Autodesk Inventor part; units mm, degrees
ref_plane "YZ Plane" through (0, 0, 0) normal (1, 0, 0) x (0, 1, 0)
ref_plane "XZ Plane" through (0, 0, 0) normal (0, 1, 0) x (-1, 0, 0)
ref_plane "XY Plane" through (0, 0, 0) normal (0, 0, 1) x (1, 0, 0)
sketch "スケッチ1" plane through (0, 0, 0) normal (0, 0, 1) x (1, 0, 0)
  line L0 (4.5, 4.5) -> (-4.5, 4.5)
  line L1 (-4.5, 4.5) -> (-4.5, -4.5)
  line L2 (-4.5, -4.5) -> (4.5, -4.5)
  line L3 (4.5, -4.5) -> (4.5, 4.5)
  line L4 (4.5, 4.5) -> (-4.5, -4.5) construction
  line L5 (-4.5, 4.5) -> (4.5, -4.5) construction
  line L6 (-3.5, 3.5) -> (3.5, 3.5)
  line L7 (3.5, 3.5) -> (3.5, -3.5)
  line L8 (3.5, -3.5) -> (-3.5, -3.5)
  line L9 (-3.5, -3.5) -> (-3.5, 3.5)
  point P0 (0, 0)
  dimension "d0" = 9
  dimension "d1" = 9
  dimension "d2" = 1
extrude "押し出し1" add sketch "スケッチ1" along normal blind 79
sketch "スケッチ2" plane through (4.5, -4.5, 0) normal (1, 0, 0) x (0, 0, -1)
  circle A0 centre (-4.5, 4.5) radius 1.6
  circle A1 centre (-74.5, 4.5) radius 1.6
  line L0 (0, 0) -> (0, 9)
  point P0 (0, 4.5)
  point P1 (0, 4.5)
  dimension "d5" = 3.2
  dimension "d6" = 3.2
  dimension "d7" = 4.5
  dimension "d8" = 70
extrude "押し出し2" cut sketch "スケッチ2" against normal through all
sketch "スケッチ3" plane through (-4.5, 4.5, 0) normal (0, 1, 0) x (1, 0, 0)
  circle A0 centre (4.5, -14.5) radius 1.6
  circle A1 centre (4.5, -64.5) radius 1.6
  line L0 (9, 0) -> (0, 0)
  point P0 (4.5, 0)
  point P1 (4.5, 0)
  dimension "d11" = 3.2
  dimension "d12" = 3.2
  dimension "d13" = 50
  dimension "d14" = 14.5
extrude "押し出し3" cut sketch "スケッチ3" against normal through all
properties part number "ハンド_角柱2" material "アルミニウム 6061"
For this review, take the finished solid that the model builds, in its own axes (mm). A direction names the side the tool comes from. Coordinates: 2 decimals unless noted, no trailing zeros. Loops run counter-clockwise (first coordinate to the right, second up) from the corner with the lowest first, then second, coordinate; pieces in that order, holes last. Notation, with made-up numbers: (-26, 3) -> (33, 3) arc R29 cw to (33, 25) -> close; hole circle Ø3 at (38, 77). An arc over 180 degrees is marked (long way). Return JSON: item names as keys, results as strings. Group by question number.
(1) For pin 1 Ø5 at (x, y) = (3, 0) entering from +Z; pin 2 Ø2.5 at (y, z) = (0, 4.5) entering from +X (3 decimals), all flat-tipped, find the tip position at first contact; note any pin that passes through.
(2) Tool access review of faces 4 (the flat face through (0, 4.5, 39)), 5 (the flat face through (0, -3.5, 39)): name each direction out of +Z, -Z, +X, -X, +Y, -Y from which nothing blocks a thin tool from reaching the whole face with its end or side.
(3) Consider section C-C, the plane y = 2.5. Give the boundary of the cut face in (x, z), plus the area to 3 significant figures.
(4) Consider section A-A, the plane x = 0. Give the boundary of the cut face in (y, z).
(5) To check wall thickness, follow L1, parallel to Z at x = 0, y = -3.95; L2, parallel to X at y = -0.25, z = 34.5. State the ranges of each line that lie inside material, in increasing order.
(6) Consider section D-D, the plane z = 64.5. Give the boundary of the cut face in (x, y).
(7) Mouldability with a two-part tool opening along Z and no side actions: class faces 1 (the flat face through (4.5, 0, 39)), 2 (the flat face through (-4, 0, 0)), 3 (the cylindrical face through (-0.208, 4.007, 62.914)) as pulls with the +Z half, pulls with the -Z half, needs draft (parallel to the pull), parting line crosses it, or undercut.
(8) Consider section B-B, the plane z = 29. Give the boundary of the cut face in (x, y), plus the area to 3 significant figures.
Results below:
{
 "1": {"pin 1": "stops at z = 79", "pin 2": "passes through"},
 "2": {"face 4": "+Z, -Z, +X, -X, +Y", "face 5": "+Z, -Z"},
 "3": {"outline": "(-4.5, 0) -> (-3.5, 0) -> (-3.5, 79) -> (-4.5, 79) -> close; (3.5, 0) -> (4.5, 0) -> (4.5, 79) -> (3.5, 79) -> close", "area": "158 mm2"},
 "4": {"outline": "(-4.5, 0) -> (-3.5, 0) -> (-3.5, 12.9) -> (-4.5, 12.9) -> close; (-4.5, 16.1) -> (-3.5, 16.1) -> (-3.5, 62.9) -> (-4.5, 62.9) -> close; (-4.5, 66.1) -> (-3.5, 66.1) -> (-3.5, 79) -> (-4.5, 79) -> close; (3.5, 0) -> (4.5, 0) -> (4.5, 12.9) -> (3.5, 12.9) -> close; (3.5, 16.1) -> (4.5, 16.1) -> (4.5, 62.9) -> (3.5, 62.9) -> close; (3.5, 66.1) -> (4.5, 66.1) -> (4.5, 79) -> (3.5, 79) -> close"},
 "5": {"L1": "z = 0 to 12.9, 16.1 to 62.9, 66.1 to 79", "L2": "x = -4.5 to -3.5, 3.5 to 4.5"},
 "6": {"outline": "(-4.5, -4.5) -> (-1.6, -4.5) -> (-1.6, -3.5) -> (-3.5, -3.5) -> (-3.5, 3.5) -> (-1.6, 3.5) -> (-1.6, 4.5) -> (-4.5, 4.5) -> close; (1.6, -4.5) -> (4.5, -4.5) -> (4.5, 4.5) -> (1.6, 4.5) -> (1.6, 3.5) -> (3.5, 3.5) -> (3.5, -3.5) -> (1.6, -3.5) -> close"},
 "7": {"face 1": "needs draft", "face 2": "pulls with the -Z half", "face 3": "undercut"},
 "8": {"outline": "(-4.5, -4.5) -> (4.5, -4.5) -> (4.5, 4.5) -> (-4.5, 4.5) -> close; hole (-3.5, -3.5) -> (3.5, -3.5) -> (3.5, 3.5) -> (-3.5, 3.5) -> close", "area": "32.0 mm2"}
}
